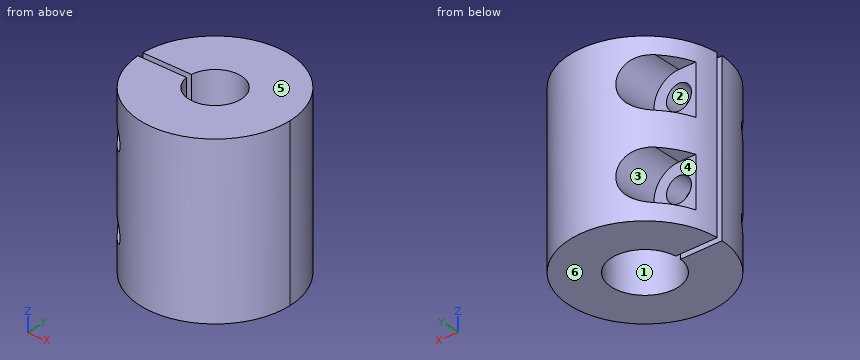
from build123d import *

# Parameters (mm, degrees)
SKETCH_1_R          = 9
EXTRUDE_1_DEPTH     = 20
SKETCH_2_R          = 3.15
CUT_EXTRUDE_1_DEPTH = 24.706539182
SKETCH_3_R          = 4
CUT_EXTRUDE_2_DEPTH = 10
SKETCH_4_W          = 11.134080052
SKETCH_4_H          = 0.7
CUT_EXTRUDE_3_DEPTH = 24.706539182
CUT_EXTRUDE_4_DEPTH = 25.928347318
SKETCH_6_R          = 1.5
CUT_EXTRUDE_5_DEPTH = 2.5
SKETCH_7_R          = 1.25
CUT_EXTRUDE_6_DEPTH = 24.841612942


with BuildPart() as part:
    # Эскиз1 → Бобышка-Вытянуть1 (new body)
    with BuildSketch(Plane.XY):
        Circle(SKETCH_1_R)
    extrude(amount=EXTRUDE_1_DEPTH)

    # Эскиз2 → Вырез-Вытянуть1 (cut, through all)
    with BuildSketch(Plane.XY.offset(20)):
        Circle(SKETCH_2_R)
    extrude(amount=-CUT_EXTRUDE_1_DEPTH, mode=Mode.SUBTRACT)

    # Эскиз3 → Вырез-Вытянуть2 (cut)
    with BuildSketch(Plane(origin=(0, 0, 0), x_dir=(-1, 0, 0), z_dir=(0, 0, -1))):
        Circle(SKETCH_3_R)
    extrude(amount=-CUT_EXTRUDE_2_DEPTH, mode=Mode.SUBTRACT)

    # Эскиз4 → Вырез-Вытянуть3 (cut, through all)
    with BuildSketch(Plane(origin=(0, 0, 0), x_dir=(-1, 0, 0), z_dir=(0, 0, -1))):
        with Locations((7.860965997, 0)):
            Rectangle(SKETCH_4_W, SKETCH_4_H)
    extrude(amount=-CUT_EXTRUDE_3_DEPTH, mode=Mode.SUBTRACT)

    # Эскиз5 → Вырез-Вытянуть4 (cut, through all)
    with BuildSketch(Plane(origin=(0, 2.85, 0), x_dir=(-1, 0, 0), z_dir=(0, -1, 0))):
        with BuildLine():
            Line((6.5, -2), (11.780255313, -2))
            Line((11.780255313, -2), (11.780255313, -8))
            Line((11.780255313, -8), (6.5, -8))
            ThreePointArc((6.5, -8), (3.5, -5), (6.5, -2))
        make_face()
        with BuildLine():
            Line((6.5, -12), (11.780255313, -12))
            Line((11.780255313, -12), (11.780255313, -18))
            Line((11.780255313, -18), (6.5, -18))
            ThreePointArc((6.5, -18), (3.5, -15), (6.5, -12))
        make_face()
    extrude(amount=-CUT_EXTRUDE_4_DEPTH, mode=Mode.SUBTRACT)

    # Эскиз6 → Вырез-Вытянуть5 (cut)
    with BuildSketch(Plane(origin=(0, 2.85, 0), x_dir=(1, 0, 0), z_dir=(0, 1, 0))):
        with Locations(Location((-6.5, -5, 0), (0, 0, 270))):
            Circle(SKETCH_6_R)
        with Locations(Location((-6.5, -15, 0), (0, 0, 270))):
            Circle(SKETCH_6_R)
    extrude(amount=-CUT_EXTRUDE_5_DEPTH, mode=Mode.SUBTRACT)

    # Эскиз7 → Вырез-Вытянуть6 (cut, through all)
    with BuildSketch(Plane(origin=(0, -0.35, 0), x_dir=(1, 0, 0), z_dir=(0, 1, 0))):
        with Locations(Location((-6.5, -5, 0), (0, 0, 270))):
            Circle(SKETCH_7_R)
        with Locations(Location((-6.5, -15, 0), (0, 0, 270))):
            Circle(SKETCH_7_R)
    extrude(amount=-CUT_EXTRUDE_6_DEPTH, mode=Mode.SUBTRACT)


solid = part.part
Input: part model. Units: mm. Frame: model coordinates. Face numbers are marked on the shaded views. A direction names the side the tool comes from. Coordinates: 2 decimals unless noted, no trailing zeros. Loops run counter-clockwise (first coordinate to the right, second up) from the corner with the lowest first, then second, coordinate; pieces in that order, holes last. Notation, with made-up numbers: (23.5, 60) -> (67.5, 60) arc R21 ccw to (67.5, 82) -> close; hole circle Ø1 at (47, -38.75). An arc over 180 degrees is marked (long way). Write item = value, one per line. Start each with the question number.
Item 1: Mould query, pull axis Z, two halves, no side actions, for the marked faces 4, 5 and 6. Classes: pulls with the +Z half, pulls with the -Z half, needs draft (parallel to the pull), parting line crosses it, or undercut.
Item 2: Reachability of the marked faces 1, 2 and 3 from +Z, -Z, +X, -X, +Y, -Y: full face, straight path, thin tool, end or side. Return the list, or none.
Item 3: Cut plane A-A, the plane y = 1.75. Return loops of the section in (x, z).
Item 4: Material intervals for line 1 (Z direction, x = -6.5, y = -5.5); line 2 (Z direction, x = -7, y = 0.75); line 3 (Y direction, x = -4.75, z = 7), sorted ascending.
Item 5: Cut plane B-B, the plane x = 0. Return loops of the section in (y, z).
Item 6: First-contact query: P1, Ø4, axis at x = -6.5, z = 15, coming from the -Y side; P2, Ø1.8, axis at x = -5, z = 14, coming from the -Y side; P3, Ø3.5, axis at x = -6.5, z = 5, coming from the +Y side; P4, Ø1.5, axis at x = -6.5, z = 15, coming from the -Y side. Flat tips, straight axial feed; report the tip coordinate or a pass-through.
Item 7: Cut plane D-D, the plane x = -4.25. Return loops of the section in (y, z).
Item 8: Cut plane C-C, the plane z = 5. Return loops of the section in (x, y).
Ans:
q1.face_4 = undercut
q1.face_5 = pulls with the +Z half
q1.face_6 = pulls with the -Z half
q2.face_1 = -Z
q2.face_2 = +Y
q2.face_3 = -X, +Y
q3.outline = (-8.83, 0) -> (-3.6, 0) -> (-3.6, 10) -> (-2.62, 10) -> (-2.62, 20) -> (-8.83, 20) -> close; (2.62, 10) -> (3.6, 10) -> (3.6, 0) -> (8.83, 0) -> (8.83, 20) -> (2.62, 20) -> close; hole circle Ø3 at (-6.5, 5); hole circle Ø3 at (-6.5, 15)
q4.line_1 = 0 to 3.75, 6.25 to 13.75, 16.25 to 20
q4.line_2 = 0 to 3.59, 6.41 to 13.59, 16.41 to 20
q4.line_3 = -7.64 to -0.35, 0.35 to 2.85
q5.outline = (-9, 0) -> (-4, 0) -> (-4, 10) -> (-3.15, 10) -> (-3.15, 20) -> (-9, 20) -> close; (3.15, 10) -> (4, 10) -> (4, 0) -> (9, 0) -> (9, 20) -> (3.15, 20) -> close
q6.P1 = -7.79
q6.P2 = -8.01
q6.P3 = 2.85
q6.P4 = through
q7.outline = (-7.93, 0) -> (-0.35, 0) -> (-0.35, 20) -> (-7.93, 20) -> close; (0.35, 0) -> (7.93, 0) -> (7.93, 3.02) -> (2.85, 3.02) -> (2.85, 6.98) -> (7.93, 6.98) -> (7.93, 13.02) -> (2.85, 13.02) -> (2.85, 16.98) -> (7.93, 16.98) -> (7.93, 20) -> (0.35, 20) -> close
q8.outline = (-8.99, -0.35) arc R9 ccw to (-7.75, -4.58) -> (-7.75, -0.35) -> close; (-8.99, 0.35) -> (-8, 0.35) -> (-8, 2.85) -> (-8.54, 2.85) arc R9 ccw to start; (-5.25, -7.31) arc R9 ccw (long way) to (-3.5, 8.29) -> (-3.5, 2.85) -> (-5, 2.85) -> (-5, 0.35) -> (-3.98, 0.35) arc R4 cw (long way) to (-3.98, -0.35) -> (-5.25, -0.35) -> close
